Check sheet for the modelled part. Datum: model origin and axes. Units: mm. A direction names the side the tool comes from. Give positions to 0.01 mm unless a question says otherwise; leave off trailing zeros. Loops run counter-clockwise (first coordinate to the right, second up) from the corner with the lowest first, then second, coordinate; pieces in that order, holes last. Notation, with made-up numbers: (-6, 22) -> (17, 22) arc R12 ccw to (17, 38) -> close; hole circle Ø4 at (33, -37). An arc over 180 degrees is marked (long way). Write each question's results on one line, items separated by ' | '. Start each with the question number.
Item 1: Scan lines: line 1 along Y through (x, z) = (42.1, -1.3); line 2 along Z through (x, y) = (19, 5); line 3 along X through (y, z) = (7.7, -0.7). Record each from-to range of solid material in increasing order.
Item 2: Cross-section at A-A on x = 10. Enter the section's corners in (y, z), then the cut area to 3 significant figures.
Item 3: Gauge pin test, flat ends, axial feed: pin 1 Ø4 at (y, z) = (24, 13) entering from -X; pin 2 Ø1.6 at (x, z) = (3.5, 15) entering from -Y; pin 3 Ø3 at (x, z) = (27, 23) entering from -Y. Record the tip position at first contact, or that the pin passes through.
Item 4: Cross-section at C-C on x = 39. Enter the section's corners in (y, z), then the cut area to 3 significant figures.
Item 5: Cross-section at D-D on y = 18.6. State how many separate pieces and enclosed holes the cut face has, then the cut area to 3 significant figures.
Item 6: Access from +Z, -Z, +X, -X, +Y, -Y to the whole of each face (thin tool, end or side, straight path). Record for faces 4 (the face through (32.7, 24, 18)), 5 (the face through (24.56, 32.96, 27.25)), 6 (the face through (3.34, 1.75, 34.49)).
Item 7: Mould release check, pull along X, two halves, no side actions. Record for faces 1 (the face through (49.7, 18, 14)), 2 (the face through (0, 19, 10)), 3 (the face through (46.36, 35.49, 34.45)): pulls with the +X half, pulls with the -X half, needs draft (parallel to the pull), parting line crosses it, or undercut.
from build123d import *

# Parameters (mm, degrees)
CROQUIS1_W              = 44.5
CROQUIS1_H              = 36.2
SALIENTE_EXTRUIR1_DEPTH = 37.2
CROQUIS2_R              = 17.028823748
SALIENTE_EXTRUIR2_DEPTH = 47.1
CROQUIS3_R              = 17.028823748
SALIENTE_EXTRUIR3_DEPTH = 1.5
REDONDEO1_R             = 3
REDONDEO2_R             = 3
CORTAR_EXTRUIR1_DEPTH   = 2.6


with BuildPart() as part:
    # Croquis1 → Saliente-Extruir1 (new body)
    with BuildSketch(Plane(origin=(0, 0, 0), x_dir=(1, 0, 0), z_dir=(0, 1, 0))):
        Polygon((0, 0), (0, -36.2), (-1.7, -36.2), (-1.7, -38.8), (49.7, -38.8), (49.7, 2.6), (-1.7, 2.6), (-1.7, 0), align=None)
        with Locations((24.85, -18.1)):
            Rectangle(CROQUIS1_W, CROQUIS1_H, mode=Mode.SUBTRACT)
    extrude(amount=SALIENTE_EXTRUIR1_DEPTH)

    # Croquis2 → Saliente-Extruir2 (add)
    with BuildSketch(Plane.ZY):
        with Locations((18.1, 18.6)):
            Circle(CROQUIS2_R)
    extrude(amount=-SALIENTE_EXTRUIR2_DEPTH)

    # Croquis3 → Saliente-Extruir3 (add)
    with BuildSketch(Plane(origin=(2.6, 0, 0), x_dir=(0, 0, -1), z_dir=(1, 0, 0))):
        with BuildLine():
            Line((-0.85, 3.85), (-0.85, 33.35))
            ThreePointArc((-0.85, 33.35), (-1.728679656, 35.471320344), (-3.85, 36.35))
            Line((-3.85, 36.35), (-32.35, 36.35))
            ThreePointArc((-32.35, 36.35), (-34.471320344, 35.471320344), (-35.35, 33.35))
            Line((-35.35, 33.35), (-35.35, 3.85))
            ThreePointArc((-35.35, 3.85), (-34.471320344, 1.728679656), (-32.35, 0.85))
            Line((-32.35, 0.85), (-3.85, 0.85))
            ThreePointArc((-3.85, 0.85), (-1.728679656, 1.728679656), (-0.85, 3.85))
        make_face()
        with Locations(Location((-18.1, 18.6, 0), (0, 0, 180))):
            Circle(CROQUIS3_R, mode=Mode.SUBTRACT)
    saliente_extruir3 = extrude(amount=SALIENTE_EXTRUIR3_DEPTH)

    # Simetría1: Saliente-Extruir3 across plane
    add(saliente_extruir3.mirror(Plane(origin=(24.85, 0, 0), x_dir=(0, 0, 1), z_dir=(1, 0, 0))))

    # Croquis4 → Cortar-Revolución1 (revolve, cut)
    with BuildSketch(Plane(origin=(0, 18.6, 0), x_dir=(1, 0, 0), z_dir=(0, 1, 0))):
        Polygon((49.7, -18.1), (0, -18.1), (0, -11.9), (32.7, -11.9), (32.7, -13.1), (36.9, -13.1), (36.9, -15.6), (49.7, -15.6), align=None)
    revolve(axis=Axis((49.7, 18.6, 18.1), (-1, 0, 0)), mode=Mode.SUBTRACT)

    # Redondeo1
    redondeo1_edges = [part.edges().sort_by_distance(p)[0] for p in [
        (49.7, 18.6, -2.6),
    ]]
    fillet(redondeo1_edges, radius=REDONDEO1_R)

    # Redondeo2
    redondeo2_edges = [part.edges().sort_by_distance(p)[0] for p in [
        (49.7, 18.6, 38.8),
    ]]
    fillet(redondeo2_edges, radius=REDONDEO2_R)

    # Croquis5 → Cortar-Extruir1 (cut)
    with BuildSketch(Plane(origin=(0, 0, -2.6), x_dir=(-1, 0, 0), z_dir=(0, 0, -1))):
        with BuildLine():
            Line((-42.1, 28), (-42.1, 29.5))
            Line((-42.1, 29.5), (-40.6, 29.5))
            ThreePointArc((-40.6, 29.5), (-43.160660172, 30.560660172), (-42.1, 28))
        make_face()
        with BuildLine():
            Line((-40.6, 29.5), (-42.1, 29.5))
            Line((-42.1, 29.5), (-42.1, 28))
            ThreePointArc((-42.1, 28), (-41.039339828, 28.439339828), (-40.6, 29.5))
        make_face()
        with BuildLine():
            ThreePointArc((-40.6, 7.7), (-41.039339828, 8.760660172), (-42.1, 9.2))
            Line((-42.1, 9.2), (-42.1, 7.7))
            Line((-42.1, 7.7), (-40.6, 7.7))
        make_face()
        with BuildLine():
            Line((-42.1, 7.7), (-42.1, 9.2))
            ThreePointArc((-42.1, 9.2), (-43.160660172, 6.639339828), (-40.6, 7.7))
            Line((-40.6, 7.7), (-42.1, 7.7))
        make_face()
        with BuildLine():
            ThreePointArc((-11.1, 7.7), (-11.539339828, 8.760660172), (-12.6, 9.2))
            Line((-12.6, 9.2), (-12.6, 7.7))
            Line((-12.6, 7.7), (-14.1, 7.7))
            ThreePointArc((-14.1, 7.7), (-12.6, 6.2), (-11.1, 7.7))
        make_face()
        with BuildLine():
            Line((-12.6, 7.7), (-12.6, 9.2))
            ThreePointArc((-12.6, 9.2), (-13.660660172, 8.760660172), (-14.1, 7.7))
            Line((-14.1, 7.7), (-12.6, 7.7))
        make_face()
        with BuildLine():
            ThreePointArc((-11.1, 29.5), (-12.6, 31), (-14.1, 29.5))
            Line((-14.1, 29.5), (-12.6, 29.5))
            Line((-12.6, 29.5), (-12.6, 28))
            ThreePointArc((-12.6, 28), (-11.539339828, 28.439339828), (-11.1, 29.5))
        make_face()
        with BuildLine():
            Line((-12.6, 29.5), (-14.1, 29.5))
            ThreePointArc((-14.1, 29.5), (-13.660660172, 28.439339828), (-12.6, 28))
            Line((-12.6, 28), (-12.6, 29.5))
        make_face()
    extrude(amount=-CORTAR_EXTRUIR1_DEPTH, mode=Mode.SUBTRACT)


solid = part.part
Answer sheet:
1) line 1: y = 0 to 6.2, 9.2 to 28, 31 to 37.2 | line 2: z = -2.6 to 0, 7.85 to 28.35, 36.2 to 38.8 | line 3: x = -1.7 to 11.1, 14.1 to 40.6, 43.6 to 49.49
2) outline: (0, -2.6) -> (37.2, -2.6) -> (37.2, 0) -> (0, 0) -> close; (0, 36.2) -> (37.2, 36.2) -> (37.2, 38.8) -> (0, 38.8) -> close; circle Ø34.06 at (18.6, 18.1); hole circle Ø12.4 at (18.6, 18.1) | area: 984 mm²
3) pin 1: stops at x = 0 | pin 2: stops at y = 0.85 | pin 3: stops at y = 1.91
4) outline: (0, -2.6) -> (37.2, -2.6) -> (37.2, 0) -> (0, 0) -> close; (0, 36.2) -> (37.2, 36.2) -> (37.2, 38.8) -> (0, 38.8) -> close; circle Ø34.06 at (18.6, 18.1); hole circle Ø5 at (18.6, 18.1) | area: 1,080 mm²
5) separate pieces: 2 | enclosed holes: 2 | area: 1,460 mm²
6) face 4: -X | face 5: none | face 6: -Y
7) face 1: pulls with the +X half | face 2: pulls with the -X half | face 3: undercut
